from build123d import *

# Parameters (mm, degrees)
F0_W     = 42
F0_H     = 65
F0_R     = 1.5
F0_R_2   = 2
F1_DEPTH = 1.25


with BuildPart() as f1:
    # F0 (on Front) → F1 (new body, symmetric)
    with BuildSketch(Plane.XZ):
        Rectangle(F0_W, F0_H)
        with Locations((-12, -8.5)):
            Circle(F0_R, mode=Mode.SUBTRACT)
        with Locations((0, -22.5)):
            Circle(F0_R_2, mode=Mode.SUBTRACT)
        with Locations((12, -8.5)):
            Circle(F0_R, mode=Mode.SUBTRACT)
        with Locations((-12, 28.4375)):
            Circle(F0_R, mode=Mode.SUBTRACT)
        with Locations((0, 15.5)):
            Circle(F0_R_2, mode=Mode.SUBTRACT)
        with Locations((12, 28.4375)):
            Circle(F0_R, mode=Mode.SUBTRACT)
    extrude(amount=F1_DEPTH, both=True)


solid = f1.part
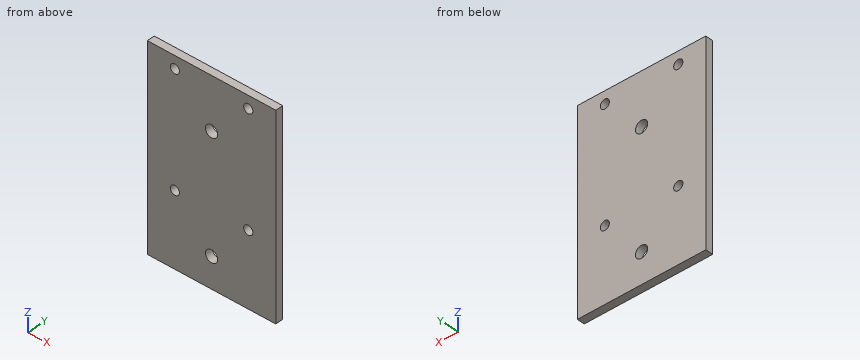
Geometry: final body of the model. Coordinates: model frame, mm. Round coordinates to 2 decimals unless told otherwise and drop trailing zeros. Loops run counter-clockwise (first coordinate to the right, second up) from the corner with the lowest first, then second, coordinate; pieces in that order, holes last.
Q1. Section C-C on z = 15.5. Return loops of the section in (x, y), plus the area to 3 significant figures.
Q2. Pin query (flat end, axial travel): P1, Ø3.5, axis at x = -12, z = 28.44, coming from the +Y side. Return the tip coordinate at first contact, or that it passes through.
Q3. Section D-D on y = -0.85. Return loops of the section in (x, z), plus the area to 3 significant figures.
Q4. Material intervals for L1, parallel to Z at x = 0, y = -0.3; L2, parallel to Z at x = 12, y = -0.65; L3, parallel to X at y = -0.4, z = 27.5, sorted ascending.
Q5. Section A-A on x = -12. Return loops of the section in (y, z).
Q6. Section B-B on z = -8.5. Return loops of the section in (x, y).
Evaluation:
1. outline: (-21, -1.25) - (-2, -1.25) - (-2, 1.25) - (-21, 1.25) - close; (2, -1.25) - (21, -1.25) - (21, 1.25) - (2, 1.25) - close
1. area: 95.0 mm2
2. P1: stops at y = 1.25
3. outline: (-21, -32.5) - (21, -32.5) - (21, 32.5) - (-21, 32.5) - close; hole circle Ø3 at (-12, -8.5); hole circle Ø3 at (-12, 28.44); hole circle Ø4 at (0, -22.5); hole circle Ø4 at (0, 15.5); hole circle Ø3 at (12, -8.5); hole circle Ø3 at (12, 28.44)
3. area: 2,680 mm2
4. L1: z = -32.5 to -24.5, -20.5 to 13.5, 17.5 to 32.5
4. L2: z = -32.5 to -10, -7 to 26.94, 29.94 to 32.5
4. L3: x = -21 to -13.17, -10.83 to 10.83, 13.17 to 21
5. outline: (-1.25, -32.5) - (1.25, -32.5) - (1.25, -10) - (-1.25, -10) - close; (-1.25, -7) - (1.25, -7) - (1.25, 26.94) - (-1.25, 26.94) - close; (-1.25, 29.94) - (1.25, 29.94) - (1.25, 32.5) - (-1.25, 32.5) - close
6. outline: (-21, -1.25) - (-13.5, -1.25) - (-13.5, 1.25) - (-21, 1.25) - close; (-10.5, -1.25) - (10.5, -1.25) - (10.5, 1.25) - (-10.5, 1.25) - close; (13.5, -1.25) - (21, -1.25) - (21, 1.25) - (13.5, 1.25) - close
